Input: part model. Units: mm. Frame: model coordinates. Face numbers are marked on the shaded views. A direction names the side the tool comes from. Round coordinates to 2 decimals unless told otherwise and drop trailing zeros. Loops run counter-clockwise (first coordinate to the right, second up) from the corner with the lowest first, then second, coordinate; pieces in that order, holes last.
(1) First-contact query: pin 1 Ø3.5 at (y, z) = (0, -1.5) entering from -X; pin 2 Ø2.5 at (x, z) = (-1, -2.5) entering from +Y; pin 3 Ø4 at (x, z) = (-2.5, -4.5) entering from -Y; pin 4 Ø1 at (x, z) = (-3.5, 0.5) entering from -Y. Flat tips, straight axial feed; report the tip coordinate or a pass-through.
(2) Cut plane B-B, the plane z = -8.75. Output: boundary loops of the cut face in (x, y), and give its area (3 significant figures).
(3) Access query for the marked faces 1, 2 and 3. Directions: +Z, -Z, +X, -X, +Y, -Y. A direction counts if a zero-diameter tool reaches every point of the face in a straight line with its end or side. Return the directions, or none.
(4) Cut plane A-A, the plane x = 0. Output: boundary loops of the cut face in (y, z), and give its area (3 significant figures).
(5) Cut plane C-C, the plane z = -1.25. Output: boundary loops of the cut face in (x, y).
(6) Line query: line 1 (Y direction, x = 0, z = 3.35); line 2 (Z direction, x = 4, y = 2); line 3 (Z direction, x = 0, y = 2.5). Output: solid intervals per line, ascending.
(7) Cut plane D-D, the plane y = -1.25. Output: boundary loops of the cut face in (x, z), and give its area (3 significant figures).
from build123d import *

# Parameters (mm, degrees)
ESQUISSE1_R             = 4.95
BOSS_EXTRU_1_DEPTH      = 2.7
ESQUISSE2_W             = 7.5
ESQUISSE2_H             = 6.5
BOSS_EXTRU_2_DEPTH      = 4.75
ESQUISSE3_R             = 4.1
BOSS_EXTRU_3_DEPTH      = 0.7
CHANFREIN1_SIZE         = 1
ESQUISSE4_R             = 0.25
BOSS_EXTRU_4_DEPTH      = 5
ENL_V_MAT_EXTRU_1_DEPTH = 0.1


with BuildPart() as part:
    # Esquisse1 → Boss.-Extru.1 (new body)
    with BuildSketch(Plane.XY):
        with Locations(Location((0, 0, 0), (0, 0, 180))):
            Circle(ESQUISSE1_R)
    extrude(amount=BOSS_EXTRU_1_DEPTH)

    # Esquisse2 → Boss.-Extru.2 (add)
    with BuildSketch(Plane(origin=(0, 0, 0), x_dir=(-1, 0, 0), z_dir=(0, 0, -1))):
        Rectangle(ESQUISSE2_W, ESQUISSE2_H)
    extrude(amount=BOSS_EXTRU_2_DEPTH)

    # Esquisse3 → Boss.-Extru.3 (add)
    with BuildSketch(Plane.XY.offset(2.7)):
        Circle(ESQUISSE3_R)
    extrude(amount=BOSS_EXTRU_3_DEPTH)

    # Chanfrein1
    # the kernel refuses this chamfer: 1 mm, written as the material it takes off along each edge
    with BuildSketch(Plane(origin=(-3.75, -3.25, 0), x_dir=(-0.027495876610586487, 0.9996219169112968, 0), z_dir=(0, 0, -1)), Plane(origin=(3.75, 3.25, 0), x_dir=(0.027495876610586487, -0.9996219169112968, 0), z_dir=(0, 0, -1)), Plane(origin=(3.75, -3.25, 0), x_dir=(-0.9996219169112968, -0.027495876610586473, 0), z_dir=(0, 0, -1))) as chanfrein1_piece_1:
        Polygon((CHANFREIN1_SIZE * 0.999621916911, CHANFREIN1_SIZE * 0.0274958766106), (-CHANFREIN1_SIZE * 0.0274958766106, CHANFREIN1_SIZE * 0.999621916911), (0, 0), align=None)
    extrude(amount=7.321682988, mode=Mode.SUBTRACT)
    with BuildSketch(Plane(origin=(-3.75, 3.25, 0), x_dir=(-0.027495876610586487, -0.9996219169112968, 0), z_dir=(0, 0, -1))) as chanfrein1_piece_2:
        Polygon((CHANFREIN1_SIZE * 0.999621916911, -CHANFREIN1_SIZE * 0.0274958766106), (-CHANFREIN1_SIZE * 0.0274958766106, -CHANFREIN1_SIZE * 0.999621916911), (0, 0), align=None)
    extrude(amount=7.321682988, mode=Mode.SUBTRACT)

    # Esquisse4 → Boss.-Extru.4 (add)
    with BuildSketch(Plane(origin=(0, 0, -4.75), x_dir=(-1, 0, 0), z_dir=(0, 0, -1))):
        with Locations((-3.25, 2.25)):
            Circle(ESQUISSE4_R)
        with Locations((0, 2.7)):
            Circle(ESQUISSE4_R)
        with Locations((3.25, 2.25)):
            Circle(ESQUISSE4_R)
        with Locations(Location((3.25, -2.25, 0), (0, 0, 180))):
            Circle(ESQUISSE4_R)
        with Locations(Location((0, -2.7, 0), (0, 0, 180))):
            Circle(ESQUISSE4_R)
        with Locations(Location((-3.25, -2.25, 0), (0, 0, 180))):
            Circle(ESQUISSE4_R)
    extrude(amount=BOSS_EXTRU_4_DEPTH)

    # Esquisse5 → Enlèv. mat.-Extru.1 (cut)
    with BuildSketch(Plane.XY.offset(3.4)):
        with BuildLine():
            Line((-0.35, 2.7), (-0.35, 0))
            ThreePointArc((-0.35, 0), (0, -0.35), (0.35, 0))
            Line((0.35, 0), (0.35, 2.7))
            ThreePointArc((0.35, 2.7), (0, 3.05), (-0.35, 2.7))
        make_face()
        with BuildLine():
            ThreePointArc((-1.325, 2.29496732), (0, -2.65), (1.325, 2.29496732))
            ThreePointArc((1.325, 2.29496732), (0.846891109, 2.166858429), (0.975, 1.688749537))
            ThreePointArc((0.975, 1.688749537), (0, -1.95), (-0.975, 1.688749537))
            ThreePointArc((-0.975, 1.688749537), (-0.846891109, 2.166858429), (-1.325, 2.29496732))
        make_face()
    extrude(amount=-ENL_V_MAT_EXTRU_1_DEPTH, mode=Mode.SUBTRACT)


solid = part.part
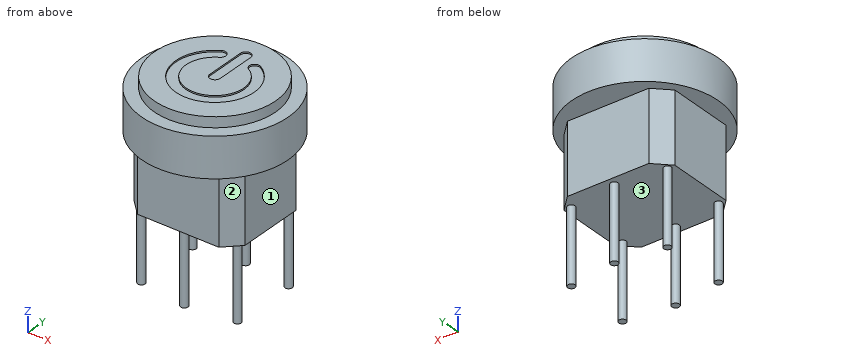
Reported:
1. pin 1: stops at x = -4.95
1. pin 2: stops at y = 3.25
1. pin 3: stops at y = -3.25
1. pin 4: stops at y = -3.94
2. outline: circle Ø0.5 at (-3.25, -2.25); circle Ø0.5 at (-3.25, 2.25); circle Ø0.5 at (0, -2.7); circle Ø0.5 at (0, 2.7); circle Ø0.5 at (3.25, -2.25); circle Ø0.5 at (3.25, 2.25)
2. area: 1.18 mm2
3. face 1: -Z, +X, +Y, -Y
3. face 2: -Z, +X, -Y
3. face 3: -Z
4. outline: (-4.95, 0) - (-3.25, 0) - (-3.25, -4.75) - (-2.95, -4.75) - (-2.95, -9.75) - (-2.45, -9.75) - (-2.45, -4.75) - (2.45, -4.75) - (2.45, -9.75) - (2.95, -9.75) - (2.95, -4.75) - (3.25, -4.75) - (3.25, 0) - (4.95, 0) - (4.95, 2.7) - (4.1, 2.7) - (4.1, 3.4) - (3.05, 3.4) - (3.05, 3.3) - (-0.35, 3.3) - (-0.35, 3.4) - (-1.95, 3.4) - (-1.95, 3.3) - (-2.65, 3.3) - (-2.65, 3.4) - (-4.1, 3.4) - (-4.1, 2.7) - (-4.95, 2.7) - close
4. area: 67.9 mm2
5. outline: (-3.75, -2.25) - (-2.75, -3.25) - (2.75, -3.25) - (3.75, -2.25) - (3.75, 2.25) - (2.75, 3.25) - (-2.75, 3.25) - (-3.75, 2.25) - close
6. line 1: y = -4.1 to -2.65, -1.95 to -0.35, 3.05 to 4.1
6. line 2: z = 0 to 2.7
6. line 3: z = -9.75 to 3.3
7. outline: (-4.79, 0) - (-3.75, 0) - (-3.75, -4.75) - (3.75, -4.75) - (3.75, 0) - (4.79, 0) - (4.79, 2.7) - (3.9, 2.7) - (3.9, 3.4) - (2.34, 3.4) - (2.34, 3.3) - (1.5, 3.3) - (1.5, 3.4) - (-1.5, 3.4) - (-1.5, 3.3) - (-2.34, 3.3) - (-2.34, 3.4) - (-3.9, 3.4) - (-3.9, 2.7) - (-4.79, 2.7) - close
7. area: 66.8 mm2
